```python
from build123d import *

# Parameters (mm, degrees)
F0_R     = 12.7
F0_R_2   = 44.45
F1_DEPTH = 6.35
F2_DEPTH = 6.35


with BuildPart() as f1:
    # F0 (on Top) → F1 (new body)
    with BuildSketch(Plane.XY):
        with BuildLine():
            ThreePointArc((-74.086042, -31.671685), (-59.255851, -34.570734), (-46.719019, -43.006782))
            ThreePointArc((-46.719019, -43.006782), (-46.143146, -43.603071), (-45.580383, -44.211748))
            ThreePointArc((-45.580383, -44.211748), (0, -63.5), (45.580383, -44.211748))
            ThreePointArc((45.580383, -44.211748), (46.143146, -43.603071), (46.719019, -43.006782))
            ThreePointArc((46.719019, -43.006782), (59.255851, -34.570734), (74.086042, -31.671685))
            ThreePointArc((74.086042, -31.671685), (75.188385, -31.694894), (76.289594, -31.74999))
            ThreePointArc((76.289594, -31.74999), (108.064688, 0), (76.289594, 31.74999))
            ThreePointArc((76.289594, 31.74999), (75.188385, 31.694894), (74.086042, 31.671685))
            ThreePointArc((74.086042, 31.671685), (59.255851, 34.570734), (46.719019, 43.006782))
            ThreePointArc((46.719019, 43.006782), (46.143146, 43.603071), (45.580383, 44.211748))
            ThreePointArc((45.580383, 44.211748), (0, 63.5), (-45.580383, 44.211748))
            ThreePointArc((-45.580383, 44.211748), (-46.143146, 43.603071), (-46.719019, 43.006782))
            ThreePointArc((-46.719019, 43.006782), (-59.255851, 34.570734), (-74.086042, 31.671685))
            ThreePointArc((-74.086042, 31.671685), (-75.188385, 31.694894), (-76.289594, 31.74999))
            ThreePointArc((-76.289594, 31.74999), (-108.064688, 0), (-76.289594, -31.74999))
            ThreePointArc((-76.289594, -31.74999), (-75.188385, -31.694894), (-74.086042, -31.671685))
        make_face()
        with Locations((-76.314688, 0)):
            Circle(F0_R, mode=Mode.SUBTRACT)
        Circle(F0_R_2, mode=Mode.SUBTRACT)
        with Locations((76.314688, 0)):
            Circle(F0_R, mode=Mode.SUBTRACT)
    extrude(amount=F1_DEPTH)

    # F0 (on Top) → F2 (join)
    with BuildSketch(Plane.XY):
        with BuildLine():
            ThreePointArc((-45.580383, -44.211748), (-46.143146, -43.603071), (-46.719019, -43.006782))
            ThreePointArc((-46.719019, -43.006782), (-46.153633, -43.612981), (-45.580383, -44.211748))
        make_face()
        with BuildLine():
            ThreePointArc((-74.086042, -31.671685), (-59.255851, -34.570734), (-46.719019, -43.006782))
            ThreePointArc((-46.719019, -43.006782), (-46.143146, -43.603071), (-45.580383, -44.211748))
            ThreePointArc((-45.580383, -44.211748), (0, -63.5), (45.580383, -44.211748))
            ThreePointArc((45.580383, -44.211748), (46.143146, -43.603071), (46.719019, -43.006782))
            ThreePointArc((46.719019, -43.006782), (59.255851, -34.570734), (74.086042, -31.671685))
            ThreePointArc((74.086042, -31.671685), (75.188385, -31.694894), (76.289594, -31.74999))
            ThreePointArc((76.289594, -31.74999), (108.064688, 0), (76.289594, 31.74999))
            ThreePointArc((76.289594, 31.74999), (75.188385, 31.694894), (74.086042, 31.671685))
            ThreePointArc((74.086042, 31.671685), (59.255851, 34.570734), (46.719019, 43.006782))
            ThreePointArc((46.719019, 43.006782), (46.143146, 43.603071), (45.580383, 44.211748))
            ThreePointArc((45.580383, 44.211748), (0, 63.5), (-45.580383, 44.211748))
            ThreePointArc((-45.580383, 44.211748), (-46.143146, 43.603071), (-46.719019, 43.006782))
            ThreePointArc((-46.719019, 43.006782), (-59.255851, 34.570734), (-74.086042, 31.671685))
            ThreePointArc((-74.086042, 31.671685), (-75.188385, 31.694894), (-76.289594, 31.74999))
            ThreePointArc((-76.289594, 31.74999), (-108.064688, 0), (-76.289594, -31.74999))
            ThreePointArc((-76.289594, -31.74999), (-75.188385, -31.694894), (-74.086042, -31.671685))
        make_face()
        with Locations((-76.314688, 0)):
            Circle(F0_R, mode=Mode.SUBTRACT)
        Circle(F0_R_2, mode=Mode.SUBTRACT)
        with Locations((76.314688, 0)):
            Circle(F0_R, mode=Mode.SUBTRACT)
        with BuildLine():
            ThreePointArc((-76.289594, -31.74999), (-75.187138, -31.729972), (-74.086042, -31.671685))
            ThreePointArc((-74.086042, -31.671685), (-75.188385, -31.694894), (-76.289594, -31.74999))
        make_face()
        with BuildLine():
            ThreePointArc((46.719019, -43.006782), (46.143146, -43.603071), (45.580383, -44.211748))
            ThreePointArc((45.580383, -44.211748), (46.153633, -43.612981), (46.719019, -43.006782))
        make_face()
        with BuildLine():
            ThreePointArc((-74.086042, 31.671685), (-75.187138, 31.729972), (-76.289594, 31.74999))
            ThreePointArc((-76.289594, 31.74999), (-75.188385, 31.694894), (-74.086042, 31.671685))
        make_face()
        with BuildLine():
            ThreePointArc((76.289594, -31.74999), (75.188385, -31.694894), (74.086042, -31.671685))
            ThreePointArc((74.086042, -31.671685), (75.187138, -31.729972), (76.289594, -31.74999))
        make_face()
        with BuildLine():
            ThreePointArc((-45.580383, 44.211748), (-46.153633, 43.612981), (-46.719019, 43.006782))
            ThreePointArc((-46.719019, 43.006782), (-46.143146, 43.603071), (-45.580383, 44.211748))
        make_face()
        with BuildLine():
            ThreePointArc((74.086042, 31.671685), (75.188385, 31.694894), (76.289594, 31.74999))
            ThreePointArc((76.289594, 31.74999), (75.187138, 31.729972), (74.086042, 31.671685))
        make_face()
        with BuildLine():
            ThreePointArc((46.719019, 43.006782), (46.153633, 43.612981), (45.580383, 44.211748))
            ThreePointArc((45.580383, 44.211748), (46.143146, 43.603071), (46.719019, 43.006782))
        make_face()
    extrude(amount=F2_DEPTH)

    # F3: F1 across plane


with BuildPart() as f1_1:
    add(f1.part)
    add(f1.part.mirror(Plane.YZ))

    # F4: F1 across plane


with BuildPart() as f1_2:
    add(f1_1.part)
    add(f1_1.part.mirror(Plane.XZ))


solid = f1_2.part
```
Here's how the part is built. I have some questions about the finished solid (model axes, mm). Coordinates: 2 decimals unless noted, no trailing zeros. Write each loop counter-clockwise with the first axis right and the second up, starting at its lowest first coordinate (ties: lowest second). Pieces come first, ordered by that corner, then holes. Notation, with made-up numbers: M -7,38.5 L 13,38.5 A20 ccw 13,66.5 Z; hole C 65,27 d7. An arc over 180 degrees is marked long. Answer as CSV lines item,"result". Start each with the question number.
Q1. Suppose I cut it at D-D, the plane y = 23. List the corners of the cut face in (x, z) for me.
Q2. If we mould it in two halves opening along Y, with no side actions, what happens to faces 1 (the cylindrical face through (-59.45, -34.49, 3.13)), 2 (the cylindrical face through (88.43, 3.81, 3.13)), 3 (the cylindrical face through (0.712, 63.496, 3.131))? For each: pulls with the +Y half, pulls with the -Y half, needs draft (parallel to the pull), parting line crosses it, or undercut.
Q3. I need wall thicknesses on probe 1 along X at (y, z) = (0, 4.25); probe 2 along Y at (x, z) = (86.5, 3.75); probe 3 along Y at (x, z) = (-71, 4). Which ranges of each line are inside material? Lowest first, please. Write a range as [from, to].
Q4. Suppose I cut it at B-B, the plane z = 3. List the corners of the cut face in (x, y) for me (3 decimals), then the cut area to 3 significant figures.
Q5. Suppose I cut it at A-A, the plane x = 0. List the corners of the cut face in (y, z) for me, then the cut area to 3 significant figures.
Q6. Will these pins go through, and if not, where does the flat tip stop? pin 1 Ø2 at (y, z) = (2, 0.5) entering from -X; pin 2 Ø2 at (x, z) = (-84, 1) entering from -Y; pin 3 Ø3 at (y, z) = (25.5, 2) entering from +X.
Q7. Suppose I cut it at C-C, the plane y = 0. List the corners of the cut face in (x, z) for me, then the cut area to 3 significant figures.
Entries:
1,outline,"M -98.2,0 L -38.04,0 L -38.04,6.35 L -98.2,6.35 Z; M 38.04,0 L 98.2,0 L 98.2,6.35 L 38.04,6.35 Z"
2,face 1,"pulls with the -Y half"
2,face 2,"undercut"
2,face 3,"pulls with the +Y half"
3,probe 1,"x = [-108.06, -89.01], [-63.61, -44.45], [44.45, 63.61], [89.01, 108.06]"
3,probe 2,"y = [-30.07, -7.59], [7.59, 30.07]"
3,probe 3,"y = [-31.78, -11.53], [11.53, 31.78]"
4,outline,"M -76.29,-31.75 A31.75 ccw -74.086,-31.672 A38.1 cw -46.719,-43.007 A63.505 ccw -45.58,-44.212 A63.5 ccw 45.58,-44.212 A63.505 ccw 46.719,-43.007 A38.1 cw 74.086,-31.672 A31.75 ccw 76.29,-31.75 A31.75 ccw 76.29,31.75 A31.75 ccw 74.086,31.672 A38.1 cw 46.719,43.007 A63.505 ccw 45.58,44.212 A63.5 ccw -45.58,44.212 A63.505 ccw -46.719,43.007 A38.1 cw -74.086,31.672 A31.75 ccw -76.29,31.75 A31.75 ccw Z; hole C -76.315,0 d25.4; hole C 0,0 d88.9; hole C 76.315,0 d25.4"
4,area,"10,800 mm²"
5,outline,"M -63.5,0 L -44.45,0 L -44.45,6.35 L -63.5,6.35 Z; M 44.45,0 L 63.5,0 L 63.5,6.35 L 44.45,6.35 Z"
5,area,"242 mm²"
6,pin 1,"stops at x = -108.05"
6,pin 2,"stops at y = -31.04"
6,pin 3,"stops at x = 97.1"
7,outline,"M -108.06,0 L -89.01,0 L -89.01,6.35 L -108.06,6.35 Z; M -63.61,0 L -44.45,0 L -44.45,6.35 L -63.61,6.35 Z; M 44.45,0 L 63.61,0 L 63.61,6.35 L 44.45,6.35 Z; M 89.01,0 L 108.06,0 L 108.06,6.35 L 89.01,6.35 Z"
7,area,"485 mm²"
